Check sheet for the modelled part. Datum: model origin and axes. Units: mm. A direction names the side the tool comes from. Give positions to 0.01 mm unless a question says otherwise; leave off trailing zeros. Loops run counter-clockwise (first coordinate to the right, second up) from the corner with the lowest first, then second, coordinate; pieces in that order, holes last. Notation, with made-up numbers: (84.25, 62.25) -> (107.25, 62.25) arc R25 ccw to (107.25, 76.25) -> close; hole circle Ø3 at (-30, -10.5). An arc over 180 degrees is marked (long way). Write each question's results on one line, items separated by ' | '. Start each with the question number.
1. Cross-section at B-B on x = 0. Record the boundary of the cut face in (y, z) (3 decimals).
2. Cross-section at C-C on y = 1. Record the boundary of the cut face in (x, z), and give its area (3 significant figures).
3. Cross-section at A-A on z = -3. Record the boundary of the cut face in (x, y), and give its area (3 significant figures).
4. Tool access check on faces 5 (the face through (-18, -3, 16.45)), 6 (the face through (12.65, 0, -5)), 7 (the face through (-18, -3, 17.21)), 8 (the face through (11.89, 0, -5)), 9 (the face through (13.95, 0, 10)). Record the directions out of +Z, -Z, +X, -X, +Y, -Y that give a thin tool (end or side, any length) a straight path to the whole face; none if there is none.
5. Mould release check, pull along X, two halves, no side actions. Record for faces 1 (the face through (0, 0, 0)), 2 (the face through (0, -8.165, 10)), 3 (the face through (-11.89, 0, -5)), 4 (the face through (-0.76, -5.785, 25.438)): +X half, -X half, draft (parallel to the pull), parting line (faces both ways), or undercut.
6. Gauge pin test, flat ends, axial feed: pin 1 Ø0.6 at (x, z) = (-19, 17) entering from -Y (3 decimals); pin 2 Ø3 at (x, z) = (5, 21) entering from +Y; pin 3 Ø3 at (y, z) = (1, -7) entering from +X. Record the tip position at first contact, or that the pin passes through.
7. Cross-section at D-D on x = -16. Record the boundary of the cut face in (y, z) (3 decimals).
8. Material ranges on L1, parallel to X at y = -4.25, z = 13; L2, parallel to Z at x = 9, y = -7; L3, parallel to X at y = -2, z = -3, recorded low to high. Write a range as from..to.
Autodesk Inventor part; units mm, degrees
ref_plane "Plan YZ" through (0, 0, 0) normal (1, 0, 0) x (0, 1, 0)
ref_plane "Plan XZ" through (0, 0, 0) normal (0, 1, 0) x (-1, 0, 0)
ref_plane "Plan XY" through (0, 0, 0) normal (0, 0, 1) x (1, 0, 0)
sketch "Esquisse1" plane through (0, 0, 0) normal (0, 0, 1) x (1, 0, 0)
  line L0 (-10.45, 8.165) -> (10.45, 8.165)
  line L1 (13.95, 4.665) -> (13.95, -4.665)
  line L2 (10.45, -8.165) -> (-10.45, -8.165)
  line L3 (-13.95, -4.665) -> (-13.95, 4.665)
  line L4 (-20.5448, 0) -> (20.5448, 0) construction
  line L5 (0, -12.4458) -> (0, 12.4458) construction
  arc A0 (-10.45, 8.165) -> (-13.95, 4.665) centre (-10.45, 4.665) ccw
  arc A1 (13.95, 4.665) -> (10.45, 8.165) centre (10.45, 4.665) ccw
  arc A2 (10.45, -8.165) -> (13.95, -4.665) centre (10.45, -4.665) ccw
  arc A3 (-13.95, -4.665) -> (-10.45, -8.165) centre (-10.45, -4.665) ccw
  point P0 (0, 0)
  point P1 (-13.95, 8.165)
  point P2 (13.95, 8.165)
  point P3 (-13.95, -8.165)
  dimension "d0" = 16.33
  dimension "d1" = 27.9
  dimension "d2" = 3.5
extrude "Extrusion1" add sketch "Esquisse1" along normal blind 19.3
sketch "Esquisse6" plane through (0, 0, 19.3) normal (0, 0, 1) x (1, 0, 0)
  circle A0 centre (0, 0) radius 5.835
  dimension "d5" = 11.67
extrude "Extrusion2" add sketch "Esquisse6" along normal blind 12.45
thread "Filetage1"
sketch "Esquisse7" plane through (0, 0, 0) normal (0, 0, -1) x (-1, 0, 0)
  line L0 (0, -11.431) -> (0, 11.431) construction
  line L1 (19.53, 0) -> (-19.53, 0) construction
  line L2 (12.65, -3.2) -> (11.89, -3.2)
  line L3 (11.89, -3.2) -> (11.89, 3.2)
  line L4 (11.89, 3.2) -> (12.65, 3.2)
  line L5 (12.65, 3.2) -> (12.65, -3.2)
  line L6 (-11.89, -3.2) -> (-12.65, -3.2)
  line L7 (-12.65, -3.2) -> (-12.65, 3.2)
  line L8 (-12.65, 3.2) -> (-11.89, 3.2)
  line L9 (-11.89, 3.2) -> (-11.89, -3.2)
  line L10 (13.95, -4.665) -> (13.95, 4.665) construction
  point P0 (0, 0)
  dimension "d10" = 1.3
  dimension "d11" = 0.76
  dimension "d12" = 6.4
extrude "Extrusion3" add sketch "Esquisse7" along normal blind 10.25
sketch "Esquisse8" plane through (-13.95, -4.665, 0) normal (-1, 0, 0) x (0, 0, 1)
  line L0 (16.45, 4.55) -> (17.21, 4.55)
  line L1 (17.21, 4.55) -> (17.21, -1.85)
  line L2 (17.21, -1.85) -> (16.45, -1.85)
  line L3 (16.45, -1.85) -> (16.45, 4.55)
  line L4 (19.3, 9.33) -> (19.3, 0) construction
  line L5 (0, -3.5) -> (19.3, -3.5)
  point P0 (0, 4.665)
  dimension "d15" = 2.85
  dimension "d16" = 0.76
  dimension "d17" = 6.4
  dimension "d18" = 1.65
extrude "Extrusion4" add sketch "Esquisse8" along normal blind 9
equation "\"d16\" = d11"
equation "\"d17\" = d12"
properties part number "P1704_002_picotte_alexandre" material "."
Geometry says:
1) outline: (-8.165, 0) -> (8.165, 0) -> (8.165, 19.3) -> (5.835, 19.3) -> (5.835, 31.75) -> (-5.835, 31.75) -> (-5.835, 19.3) -> (-8.165, 19.3) -> close
2) outline: (-13.95, 0) -> (-12.65, 0) -> (-12.65, -10.25) -> (-11.89, -10.25) -> (-11.89, 0) -> (11.89, 0) -> (11.89, -10.25) -> (12.65, -10.25) -> (12.65, 0) -> (13.95, 0) -> (13.95, 19.3) -> (5.75, 19.3) -> (5.75, 31.75) -> (-5.75, 31.75) -> (-5.75, 19.3) -> (-13.95, 19.3) -> close | area: 697 mm^2
3) outline: (-12.65, -3.2) -> (-11.89, -3.2) -> (-11.89, 3.2) -> (-12.65, 3.2) -> close; (11.89, -3.2) -> (12.65, -3.2) -> (12.65, 3.2) -> (11.89, 3.2) -> close | area: 9.73 mm^2
4) face 5: -Z, -X, +Y, -Y | face 6: -Z, +X, +Y, -Y | face 7: +Z, -X, +Y, -Y | face 8: -Z, +Y, -Y | face 9: +Z, -Z, +X, +Y, -Y
5) face 1: undercut | face 2: draft | face 3: undercut | face 4: parting line
6) pin 1: y = -6.515 | pin 2: y = 4.67 | pin 3: x = 12.65
7) outline: (-6.515, 16.45) -> (-0.115, 16.45) -> (-0.115, 17.21) -> (-6.515, 17.21) -> close
8) L1: -13.95..13.95 | L2: 0..19.3 | L3: -12.65..-11.89, 11.89..12.65
